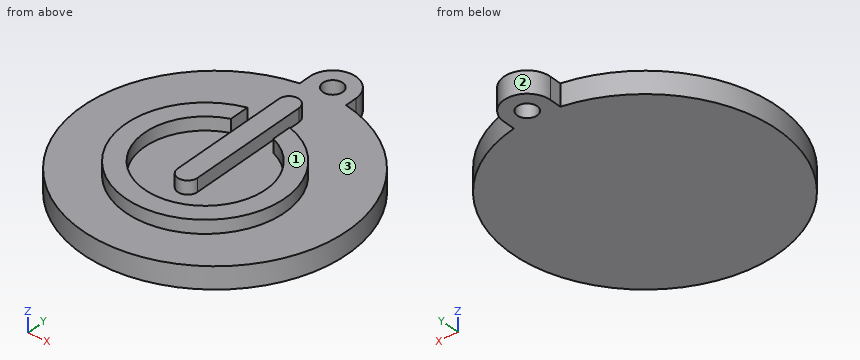
```python
from build123d import *

# Parameters (mm, degrees)
EXTRUDE_DEPTH = 3.3
SKETCH001_R   = 1.5
POCKET_DEPTH  = 3.301
PAD_DEPTH     = 2


with BuildPart() as part:
    # Sketch → Extrude (new body)
    with BuildSketch(Plane.XY):
        with BuildLine():
            ThreePointArc((3.5, 21.5), (0, 25), (-3.5, 21.5))
            Line((-3.5, 21.5), (-3.5, 19.691369))
            ThreePointArc((-3.5, 19.691369), (0, -20), (3.5, 19.691369))
            Line((3.5, 19.691369), (3.5, 21.5))
        make_face()
    extrude(amount=EXTRUDE_DEPTH)

    # Sketch001 → Pocket (cut, through all)
    with BuildSketch(Plane.XY.offset(3.3)):
        with Locations((0, 21.5)):
            Circle(SKETCH001_R)
    extrude(amount=-POCKET_DEPTH, mode=Mode.SUBTRACT)

    # Sketch002 → Pad (new body)
    with BuildSketch(Plane.XY.offset(3.3)):
        with BuildLine():
            ThreePointArc((1.5, 13.500001), (0, 15), (-1.5, 13.5))
            Line((-1.5, 13.5), (-1.5, -5))
            ThreePointArc((-1.5, -5), (0, -6.5), (1.5, -4.999999))
            Line((1.5, 13.500001), (1.5, -4.999999))
        make_face()
        with BuildLine():
            Line((-3.2, 6.765466), (-3.2, 9.765466))
            ThreePointArc((-3.2, 9.765466), (0, -13.8), (3.2, 9.765466))
            Line((3.2, 6.765466), (3.2, 9.765466))
            ThreePointArc((-3.2, 6.765466), (0, -10.943698), (3.2, 6.765466))
        make_face()
    extrude(amount=PAD_DEPTH)


solid = part.part
```
Model file for the job. Use its own axes, mm. Face numbers are marked on the shaded views. Round coordinates to 2 decimals unless told otherwise and drop trailing zeros. Order: outer loops, then holes, each group sorted by start corner. A loop starts at its lowest first (then second) coordinate and runs counter-clockwise, first axis right, second up. Notation, with made-up numbers: (-8, 77.25) -> (38, 77.25) arc R31 ccw to (38, 110.25) -> close; hole circle Ø4 at (35, 2.25). An arc over 180 degrees is marked (long way). Use one line per item in the form item = value.
Item 1: Flat gauge pins, fed straight in: pin 1 Ø0.6 at (y, z) = (3.5, 4.5) entering from -X; pin 2 Ø2 at (y, z) = (-4, 1) entering from -X; pin 3 Ø1 at (y, z) = (-10.5, 3.5) entering from +X. Where does each tip first touch, or does it go through?
Returned:
pin_1 = -10.91
pin_2 = -19.77
pin_3 = 17.3
Item 2: Pull direction X, two halves, no side cores. Call the marked faces 1, 2 and 3: released by +X, released by -X, zero draft, split by the parting line, or undercut.
Returned:
face_1 = zero draft
face_2 = split by the parting line
face_3 = undercut
Item 3: Cut at B-B, the plane z = 4.8. Write the cut outline in (x, y).
Returned:
outline = (-3.2, 6.77) -> (-3.2, 9.77) arc R12 ccw (long way) to (3.2, 9.77) -> (3.2, 6.77) arc R9.14 cw (long way) to start; (-1.5, -5) arc R1.5 ccw to (1.5, -5) -> (1.5, 13.5) arc R1.5 ccw to (-1.5, 13.5) -> close
Item 4: Cut at C-C, the plane z = 1.6. Write the cut outline in (x, y).
Returned:
outline = (-3.5, 19.69) arc R20 ccw (long way) to (3.5, 19.69) -> (3.5, 21.5) arc R3.5 ccw to (-3.5, 21.5) -> close; hole circle Ø3 at (0, 21.5)
Item 5: Cut at A-A, the plane x = 0. Write the cut outline in (y, z), and give its area (3 significant figures).
Returned:
outline = (-20, 0) -> (20, 0) -> (20, 3.3) -> (15, 3.3) -> (15, 5.3) -> (-6.5, 5.3) -> (-6.5, 3.3) -> (-10.94, 3.3) -> (-10.94, 5.3) -> (-13.8, 5.3) -> (-13.8, 3.3) -> (-20, 3.3) -> close; (23, 0) -> (25, 0) -> (25, 3.3) -> (23, 3.3) -> close
area = 187 mm^2
Item 6: Cut at D-D, the plane y = -1.8. Write the cut outline in (x, z).
Returned:
outline = (-19.92, 0) -> (19.92, 0) -> (19.92, 3.3) -> (12, 3.3) -> (12, 5.3) -> (9.14, 5.3) -> (9.14, 3.3) -> (1.5, 3.3) -> (1.5, 5.3) -> (-1.5, 5.3) -> (-1.5, 3.3) -> (-9.14, 3.3) -> (-9.14, 5.3) -> (-12, 5.3) -> (-12, 3.3) -> (-19.92, 3.3) -> close
Item 7: Drill centre lines: line 1 (X direction, y = -1.8, z = 4); line 2 (Y direction, x = 0, z = 1.15); line 3 (X direction, y = 6.5, z = 3.55). Where is each one in solid material? Low to high.
Returned:
line_1 = -12 to -9.14, -1.5 to 1.5, 9.14 to 12
line_2 = -20 to 20, 23 to 25
line_3 = -8.67 to -3.84, -1.5 to 1.5, 3.84 to 8.67
